from build123d import *

# Parameters (mm, degrees)
SKETCH2_R           = 2.5
BOSS_EXTRUDE1_DEPTH = 65
CHAMFER1_SIZE       = 0.5
CUT_EXTRUDE1_DEPTH  = 2.3
SKETCH8_R           = 1.782050808
CUT_EXTRUDE2_DEPTH  = 1
CUT_EXTRUDE2_TAPER  = 45


with BuildPart() as part:
    # Sketch2 → Boss-Extrude1 (new body)
    with BuildSketch(Plane(origin=(0, 0, 0), x_dir=(0, 0, -1), z_dir=(1, 0, 0))):
        Circle(SKETCH2_R)
    extrude(amount=-BOSS_EXTRUDE1_DEPTH)

    # Chamfer1
    chamfer1_edges = [part.edges().sort_by_distance(p)[0] for p in [
        (0, 0, 2.5),
    ]]
    chamfer(chamfer1_edges, length=CHAMFER1_SIZE)

    # Sketch6 → Revolve1 (revolve)
    with BuildSketch(Plane.XY):
        with BuildLine():
            Line((-66.5, 0), (-66.5, 4.161437828))
            ThreePointArc((-66.5, 4.161437828), (-65.75, 4.5), (-65, 4.161437828))
            Line((-65, 4.161437828), (-65, 0))
            Line((-65, 0), (-66.5, 0))
        make_face()
    revolve(axis=Axis((-65, 0, 0), (1, 0, 0)))

    # Sketch7 → Cut-Extrude1 (cut)
    with BuildSketch(Plane.ZY.offset(66.5)):
        Polygon((0, 1.732050808), (-1.5, 0.866025404), (-1.5, -0.866025404), (0, -1.732050808), (1.5, -0.866025404), (1.5, 0.866025404), align=None)
    extrude(amount=-CUT_EXTRUDE1_DEPTH, mode=Mode.SUBTRACT)

    # Sketch8 → Cut-Extrude2 (cut)
    with BuildSketch(Plane.ZY.offset(66.5)):
        Circle(SKETCH8_R)
    extrude(amount=-CUT_EXTRUDE2_DEPTH, taper=CUT_EXTRUDE2_TAPER, mode=Mode.SUBTRACT)


solid = part.part
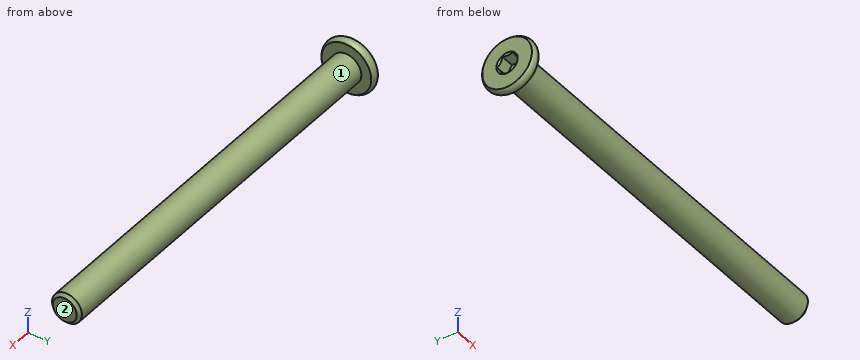
Check sheet for the modelled part. Datum: model origin and axes. Units: mm. Face numbers are marked on the shaded views. A direction names the side the tool comes from. Round coordinates to 2 decimals unless told otherwise and drop trailing zeros. Write each loop counter-clockwise with the first axis right and the second up, starting at its lowest first coordinate (ties: lowest second). Pieces come first, ordered by that corner, then holes. Notation, with made-up numbers: (52, 8) - (102, 8) arc R18 ccw to (102, 43) - close; hole circle Ø5 at (37, 72). An arc over 180 degrees is marked (long way). Return JSON: item names as keys, results as strings.
Q1. Depth check by flat-ended pin: P1, Ø0.9, axis at x = -65, y = 0, coming from the -Z side; P2, Ø2, axis at y = 3, z = 3, coming from the +X side; P3, Ø0.5, axis at x = -65, y = 0.5, coming from the +Z side. Enter the tip coordinate at first touch or a pass-through.
Returned:
{"P1": "stops at z = -4.45", "P2": "stops at x = -65", "P3": "stops at z = 4.34"}
Q2. Scan lines: L1, parallel to Y at x = -63, z = 2; L2, parallel to Z at x = -63, y = 1.75; L3, parallel to Y at x = -49, z = -0.25. Record each from-to range of solid material in increasing order. Write a range as from..to.
Returned:
{"L1": "y = -1.5..1.5", "L2": "z = -1.79..1.79", "L3": "y = -2.49..2.49"}
Q3. Cross-section at A-A (x = -30.5). Record the boundary of the cut face in (y, z), then the cut area to 3 significant figures.
Returned:
{"outline": "circle Ø5 at (0, 0)", "area": "19.6 mm²"}
Q4. Access from +Z, -Z, +X, -X, +Y, -Y to the whole of each face (thin tool, end or side, straight path). Record for the marked faces 1 and 2.
Returned:
{"face 1": "+X", "face 2": "+Z, -Z, +X, +Y, -Y"}
